Input: part model. Units: mm. Frame: model coordinates. A direction names the side the tool comes from. Give positions to 0.01 mm unless a question says otherwise; leave off trailing zeros. Loops run counter-clockwise (first coordinate to the right, second up) from the corner with the lowest first, then second, coordinate; pieces in that order, holes last. Notation, with made-up numbers: M 6,-12.5 L 23,-12.5 A26 cw 23,21.5 Z; hole C 78,78 d10. An arc over 180 degrees is marked long. Answer as a JSON object with one key per item and string values. Group by question number.
```python
from build123d import *

# Parameters (mm, degrees)
SKETCH_1_R           = 19.75
SKETCH_1_R_2         = 18.77
EXTRUDE_1_DEPTH      = 1
SKETCH_2_R           = 19.75
EXTRUDE_2_DEPTH      = 6
SKETCH_5_R           = 1.35
SKETCH_5_R_2         = 10
CUT_EXTRUDE_2_DEPTH  = 29.567901568
SKETCH_6_R           = 1.98
EXTRUDE_4_DEPTH      = 1
EXTRUDE_START        = -3
SKETCH_11_W          = 60
SKETCH_11_H          = 40
SKETCH_11_R          = 19.75
EXTRUDE_6_DEPTH      = 3
SKETCH_7_R           = 3
CUT_EXTRUDE_7_DEPTH  = 20
EXTRUDE_7_DEPTH      = 1
EXTRUDE_7_DEPTH_BACK = 2


with BuildPart() as part:
    # 草图1 → 凸台-拉伸1 (new body)
    with BuildSketch(Plane(origin=(0, 0, 0), x_dir=(1, 0, 0), z_dir=(0, 1, 0))):
        with Locations(Location((0, 0, 0), (0, 0, 270))):
            Circle(SKETCH_1_R)
        with Locations(Location((0, 0, 0), (0, 0, 270))):
            Circle(SKETCH_1_R_2, mode=Mode.SUBTRACT)
    extrude(amount=EXTRUDE_1_DEPTH)

    # 草图2 → 凸台-拉伸2 (add)
    with BuildSketch(Plane(origin=(0, 1, 0), x_dir=(1, 0, 0), z_dir=(0, 1, 0))):
        with Locations(Location((0, 0, 0), (0, 0, 270))):
            Circle(SKETCH_2_R)
    extrude(amount=EXTRUDE_2_DEPTH)

    # 草图5 → 切除-拉伸2 (cut, through all)
    with BuildSketch(Plane.XZ.offset(-1)):
        with Locations(Location((0, 13.5, 0), (0, 0, 270))):
            Circle(SKETCH_5_R)
        with Locations(Location((11.691342951, 6.75, 0), (0, 0, 270))):
            Circle(SKETCH_5_R)
        with Locations(Location((11.691342951, -6.75, 0), (0, 0, 270))):
            Circle(SKETCH_5_R)
        with Locations(Location((0, -13.5, 0), (0, 0, 270))):
            Circle(SKETCH_5_R)
        with Locations(Location((-11.691342951, -6.75, 0), (0, 0, 270))):
            Circle(SKETCH_5_R)
        with Locations(Location((-11.691342951, 6.75, 0), (0, 0, 270))):
            Circle(SKETCH_5_R)
        with Locations(Location((0, 0, 0), (0, 0, 270))):
            Circle(SKETCH_5_R_2)
    extrude(amount=-CUT_EXTRUDE_2_DEPTH, mode=Mode.SUBTRACT)

    # 草图6 → 凸台-拉伸4 (add)
    with BuildSketch(Plane.XZ.offset(-1)):
        with Locations(Location((12, 0, 0), (0, 0, 90))):
            Circle(SKETCH_6_R)
        with Locations(Location((-6, -10.392304845, 0), (0, 0, 90))):
            Circle(SKETCH_6_R)
        with Locations(Location((-6, 10.392304845, 0), (0, 0, 90))):
            Circle(SKETCH_6_R)
    extrude(amount=EXTRUDE_4_DEPTH)

    # 草图11 → 凸台-拉伸6 (add)
    with BuildSketch(Plane(origin=(0, 7, 0), x_dir=(1, 0, 0), z_dir=(0, 1, 0)).offset(EXTRUDE_START)):
        Rectangle(SKETCH_11_W, SKETCH_11_H)
        with Locations(Location((0, 0, 0), (0, 0, 270))):
            Circle(SKETCH_11_R, mode=Mode.SUBTRACT)
    extrude(amount=EXTRUDE_6_DEPTH)

    # 草图7 → 切除-拉伸7 (cut)
    with BuildSketch(Plane.XZ.offset(-1)):
        with Locations(Location((-14, 0, 0), (0, 0, 270))):
            Circle(SKETCH_7_R)
        with Locations(Location((7, 12.124355653, 0), (0, 0, 270))):
            Circle(SKETCH_7_R)
        with Locations(Location((7, -12.124355653, 0), (0, 0, 270))):
            Circle(SKETCH_7_R)
    extrude(amount=-CUT_EXTRUDE_7_DEPTH, mode=Mode.SUBTRACT)

    # 草图15 → 凸台-拉伸7 (add, two sides: drawn at the far end of the back side and taken through both)
    with BuildSketch(Plane(origin=(0, 1, 0), x_dir=(-1, 0, 0), z_dir=(0, -1, 0)).offset(-EXTRUDE_7_DEPTH_BACK)):
        with BuildLine():
            Line((-5.518906371, 18.541790589), (-5.99084035, 20.127340408))
            ThreePointArc((-5.99084035, 20.127340408), (0, 21), (5.99084035, 20.127340408))
            Line((5.99084035, 20.127340408), (5.518906371, 18.541790589))
            ThreePointArc((5.518906371, 18.541790589), (0, 19.345705616), (-5.518906371, 18.541790589))
        make_face()
    extrude(amount=EXTRUDE_7_DEPTH + EXTRUDE_7_DEPTH_BACK)


solid = part.part
```
1. Section A-A (z = 7.5). Output: boundary loops of the cut face in (x, y), then the cut area to 3 significant figures.
2. Mould query, pull axis X, two halves, no side actions, for faces 4 (the flat face through (0, 3, -20)), 5 (the cylindrical face through (0, 2, -21)), 6 (the cylindrical face through (-9.76, 3.96, 2.17)). Classes: pulls with the +X half, pulls with the -X half, needs draft (parallel to the pull), parting line crosses it, or undercut.
3. Reachability of faces 1 (the flat face through (-5.815, 1.521, -19.537)), 2 (the flat face through (5.81, 1.52, -19.52)), 3 (the cylindrical face through (-5.242, 0.507, -8.563)) from +Z, -Z, +X, -X, +Y, -Y: full face, straight path, thin tool, end or side. Return the list, or none.
4. Section B-B (x = 8). Output: boundary loops of the cut face in (y, z).
5. Material intervals for L1, parallel to X at y = 3.5, z = 0; L2, parallel to X at y = 6, z = 12; L3, parallel to X at y = 3.15, z = -6.75, sorted ascending.
6. First-contact query: P1, Ø1.5, axis at x = 9.5, z = 10.5, coming from the -Y side; P2, Ø1.5, axis at y = 1.5, z = 5, coming from the +X side; P3, Ø1, axis at x = -9.5, y = 5.5, coming from the -Z side. Flat tips, straight axial feed; report the tip coordinate or a pass-through.
7. Section C-C (z = 13). Output: boundary loops of the cut face in (x, y), then the cut area to 3 significant figures.
8. Section D-D (y = 6). Count the separate pieces of the cut face and the enclosed holes in it, then the cut area to 3 significant figures.
Geometry results:
{
 "1": {"outline": "M -30,4 L -18.27,4 L -18.27,0 L -17.21,0 L -17.21,1 L -12.81,1 L -12.81,7 L -30,7 Z; M -10.57,1 L -6.61,1 L -6.61,7 L -10.57,7 Z; M 6.61,1 L 10.57,1 L 10.57,7 L 6.61,7 Z; M 12.81,1 L 17.21,1 L 17.21,0 L 18.27,0 L 18.27,4 L 30,4 L 30,7 L 12.81,7 Z", "area": "185 mm2"},
 "2": {"face 4": "needs draft", "face 5": "parting line crosses it", "face 6": "undercut"},
 "3": {"face 1": "-X, -Y", "face 2": "+X, -Y", "face 3": "-Y"},
 "4": {"outline": "M 0,-18.06 L 4,-18.06 L 4,-20 L 7,-20 L 7,-14.95 L 1,-14.95 L 1,-16.98 L 0,-16.98 Z; M 0,16.98 L 1,16.98 L 1,14.95 L 7,14.95 L 7,20 L 4,20 L 4,18.06 L 0,18.06 Z; M 1,-9.3 L 7,-9.3 L 7,-6 L 1,-6 Z; M 1,6 L 7,6 L 7,9.3 L 1,9.3 Z"},
 "5": {"L1": "-19.75 to -17, -11 to -10, 10 to 19.75", "L2": "-30 to 4, 10 to 30", "L3": "-18.56 to -13.04, -10.34 to -7.38, 7.38 to 10.34, 13.04 to 18.56"},
 "6": {"P1": "y = 1", "P2": "x = 19.29", "P3": "z = -20"},
 "7": {"outline": "M -30,4 L -14.87,4 L -14.87,0 L -13.54,0 L -13.54,1 L -1.25,1 L -1.25,7 L -30,7 Z; M 1.25,1 L 4.13,1 L 4.13,7 L 1.25,7 Z; M 9.87,1 L 13.54,1 L 13.54,0 L 14.87,0 L 14.87,4 L 30,4 L 30,7 L 9.87,7 Z", "area": "222 mm2"},
 "8": {"separate pieces": "1", "enclosed holes": "10", "area": "1,970 mm2"}
}
